Verification items for this drawing (mm, ordinates from the low corner). A direction names the side the tool comes from. Give positions to 0.01 mm unless a question says otherwise; leave off trailing zeros. Loops run counter-clockwise (first coordinate to the right, second up) from the corner with the lowest first, then second, coordinate; pieces in that order, holes last. Notation, with made-up numbers: (65, 67) -> (119, 67) arc R5 cw to (119, 71) -> close; hole circle Ø10 at (-36.75, -8). An arc over 180 degrees is marked (long way). Answer as a JSON object with one key per item and string values.
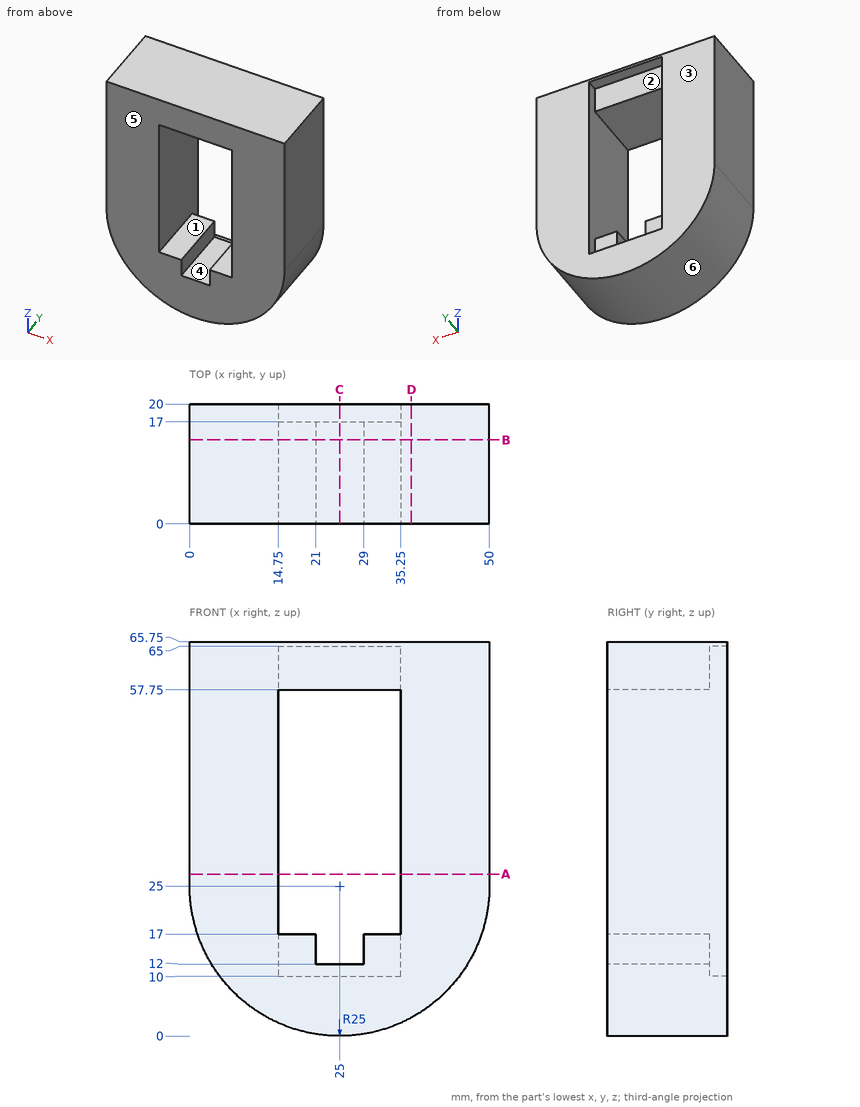
1) Section check A-A on z = 27. Record the cut outline in (x, y), plus the area to 3 significant figures.
Geometry check:
{"outline": "(0, 0) -> (14.75, 0) -> (14.75, 20) -> (0, 20) -> close; (35.25, 0) -> (50, 0) -> (50, 20) -> (35.25, 20) -> close", "area": "590 mm2"}
2) Section check D-D on x = 37. Record the cut outline in (y, z).
Geometry check:
{"outline": "(0, 3.07) -> (20, 3.07) -> (20, 65.75) -> (0, 65.75) -> close"}
3) Material ranges on line 1 along X through (y, z) = (10.25, 40); line 2 along Z through (x, y) = (24, 7.25); line 3 along X through (y, z) = (9.25, 16), recorded low to high. Write a range as from..to.
Geometry check:
{"line 1": "x = 0..14.75, 35.25..50", "line 2": "z = 0.02..12, 57.75..65.75", "line 3": "x = 1.68..21, 29..48.32"}
4) Draft check along X on the marked faces 4, 5 and 6. Enter one of: pulls with the +X half, pulls with the -X half, needs draft (parallel to the pull), parting line crosses it, or undercut.
Geometry check:
{"face 4": "undercut", "face 5": "needs draft", "face 6": "parting line crosses it"}
5) Section check C-C on x = 25. Record the cut outline in (y, z), plus the area to 3 significant figures.
Geometry check:
{"outline": "(0, 0) -> (20, 0) -> (20, 10) -> (17, 10) -> (17, 12) -> (0, 12) -> close; (0, 57.75) -> (17, 57.75) -> (17, 65) -> (20, 65) -> (20, 65.75) -> (0, 65.75) -> close", "area": "372 mm2"}
6) Depth check by flat-ended pin: P1, Ø3.5, axis at x = 26.5, y = 18.5, coming from the -Z side; P2, Ø5.5, axis at y = 10, z = 14, coming from the +X side; P3, Ø2.5, axis at y = 7, z = 13.5, coming from the -X side. Enter the tip coordinate at first touch or a pass-through.
Geometry check:
{"P1": "stops at z = 0", "P2": "stops at x = 48.6", "P3": "stops at x = 2.2"}
7) Section check B-B on y = 14. Record the cut outline in (x, z), plus the area to 3 significant figures.
Geometry check:
{"outline": "(0, 25) arc R25 ccw to (50, 25) -> (50, 65.75) -> (0, 65.75) -> close; hole (14.75, 17) -> (21, 17) -> (21, 12) -> (29, 12) -> (29, 17) -> (35.25, 17) -> (35.25, 57.75) -> (14.75, 57.75) -> close", "area": "2,140 mm2"}
8) Tool access check on the marked faces 1, 2 and 3. Record the directions out of +Z, -Z, +X, -X, +Y, -Y that give a thin tool (end or side, any length) a straight path to the whole face; none if there is none.
Geometry check:
{"face 1": "+Y, -Y", "face 2": "+Y", "face 3": "+Z, -Z, +X, -X, +Y"}
